Autodesk Inventor part; units mm, degrees
ref_plane "YZ Plane" through (0, 0, 0) normal (1, 0, 0) x (0, 1, 0)
ref_plane "XZ Plane" through (0, 0, 0) normal (0, 1, 0) x (-1, 0, 0)
ref_plane "XY Plane" through (0, 0, 0) normal (0, 0, 1) x (1, 0, 0)
sketch "Szkic1" plane through (0, 0, 0) normal (0, 0, 1) x (1, 0, 0)
  line L0 (-47.736, 26.7667) -> (-47.736, 6.7667)
  line L1 (-47.736, 26.7667) -> (52.264, 26.7667)
  line L2 (52.264, 26.7667) -> (52.264, 6.7667)
  line L3 (52.264, 6.7667) -> (32.264, 6.7667)
  line L4 (32.264, 6.7667) -> (32.264, -48.2333)
  line L5 (32.264, -48.2333) -> (-27.736, -48.2333)
  line L6 (-27.736, -48.2333) -> (-27.736, 6.7667)
  line L7 (-27.736, 6.7667) -> (-47.736, 6.7667)
  circle A0 centre (2.264, -27.7333) radius 19
  arc A1 (-11.0025, -7.7333) -> (-11.0025, -47.7333) centre (2.264, -27.7333) ccw
  line L8 (-11.0025, -47.7333) -> (15.5305, -47.7333)
  arc A2 (15.5305, -47.7333) -> (15.5305, -7.7333) centre (2.264, -27.7333) ccw
  line L9 (15.5305, -7.7333) -> (-11.0025, -7.7333)
  circle A3 centre (2.264, -27.7333) radius 15
  circle A4 centre (-37.736, 16.7667) radius 2
  circle A5 centre (2.264, 16.7667) radius 2
  circle A6 centre (42.264, 16.7667) radius 2
  arc A7 (-23.5765, -30.609) -> (-13.7282, -48.2333) centre (2.264, -27.7333) ccw
  arc A8 (18.2561, -48.2333) -> (28.1044, -30.609) centre (2.264, -27.7333) ccw
  line L10 (-27.736, 6.7667) -> (-23.5765, -30.609)
  line L11 (32.264, 6.7667) -> (28.1044, -30.609)
  line L12 (-7.736, 26.7667) -> (-7.736, 66.7667)
  line L13 (-7.736, 66.7667) -> (12.264, 66.7667)
  line L14 (12.264, 66.7667) -> (12.264, 26.7667)
  circle A9 centre (2.264, 56.7667) radius 2
  point P0 (0, 0)
  point P1 (-16.736, -27.7333)
  point P2 (-11.1711, -41.1683)
  point P3 (15.699, -14.2982)
  point P4 (15.699, -41.1683)
  point P5 (-11.1711, -14.2982)
  point P6 (21.264, -27.7333)
  dimension "d0" = 20
  dimension "d1" = 100
  dimension "d2" = 20
  dimension "d3" = 60
  dimension "d4" = 20
  dimension "d5" = 55
  dimension "d8" = 38
  dimension "d13" = 34.5
  dimension "d14" = 30
  dimension "d15" = 30
  dimension "d24" = 4
  dimension "d25" = 4
  dimension "d26" = 4
  dimension "d29" = 10
  dimension "d30" = 10
  dimension "d31" = 10
  dimension "d32" = 10
  dimension "d33" = 10
  dimension "d34" = 50
  dimension "d42" = 2
  dimension "d47" = 40
  dimension "d48" = 20
  dimension "d49" = 40
  dimension "d50" = 10
  dimension "d51" = 10
  dimension "d52" = 4
extrude "Wyciągnięcie proste1" add sketch "Szkic1" along normal blind 4 contours L1 L2 L3 L11 A8 L5 A7 L10 L7 L0 | L12 L13 L14 L1 | L10 A7 L5 L6 | A8 L11 L4 L5 | A0 | L9 A2 L8 A1 | A3 | A4 | A5 | A6 | A9
extrude "Wyciągnięcie proste2" cut sketch "Szkic1" along normal through all contours A3 | A4 | A5 | A6 | A9
hole "Otwór1" at (2.264, -27.7333, 0) at (21.264, -27.7333, 0) at (-11.1711, -41.1683, 0) at (15.699, -41.1683, 0) at (15.699, -14.2982, 0) at (-11.1711, -14.2982, 0) at (-16.736, -27.7333, 0) direction (0, 0, 1) diameter 5 end through all
extrude "Wyciągnięcie proste3" cut sketch "Szkic1" along normal blind 10 contours L10 A7 L5 L6 | A8 L11 L4 L5
fillet "Zaokrąglenie1" radius 6 8 edges at (-47.736, 6.7667, 2) (-47.736, 26.7667, 2) (52.264, 6.7667, 2) (52.264, 26.7667, 2) (-7.736, 26.7667, 2) (-7.736, 66.7667, 2) (12.264, 26.7667, 2) (12.264, 66.7667, 2)
fillet "Zaokrąglenie2" radius 10 2 edges at (-27.736, 6.7667, 2) (32.264, 6.7667, 2)
fillet "Zaokrąglenie3" radius 8 2 edges at (-13.7282, -48.2333, 2) (18.2561, -48.2333, 2)
equation "\"d2\" = -0.5 * d3 + 0.5 * d1"
equation "\"d34\" = 0.5 * d1"
properties part number "LC_ALU_4mm_Heatbed_Frame_Ball_Screw_Nut_Mounting_Bracket"
Could you check a few things on this model? Use its own coordinates, in mm. A direction names the side the tool comes from. Give positions to 0.01 mm unless a question says otherwise; leave off trailing zeros. Order: outer loops, then holes, each group sorted by start corner. A loop starts at its lowest first (then second) coordinate and runs counter-clockwise, first axis right, second up. Notation, with made-up numbers: (89.25, 25.5) - (109.25, 25.5) arc R12 ccw to (109.25, 41.5) - close; hole circle Ø5 at (-25, -35.75). An arc over 180 degrees is marked (long way). Return JSON: item names as keys, results as strings. Group by question number.
Q1. Thinking about a two-plate mould opening in X: for faces 1 (the face through (52.264, 17, 2)), 2 (the face through (-28, 26.767, 2)), 3 (the face through (-0.99, -13.09, 1.97)), 4 (the face through (3.19, 58.54, 1.97)), which applies, pulls with the +X half, pulls with the -X half, needs draft (parallel to the pull), parting line crosses it, or undercut?
Q2. Which directions (+Z, -Z, +X, -X, +Y, -Y) give clear straight access to the entire face, cutting with the end or side of a thin tool? Please do faces 5 (the face through (-39.323, 17.984, 1.972)), 6 (the face through (44, 6.767, 2)), 7 (the face through (-7.736, 47, 2)).
Q3. Suppose I cut it at B-B, the plane x = 8.5. Please give me the cut outline in (y, z), and give its area (3 significant figures).
Q4. Will these pins go through, and if not, where does the flat tip stop? pin 1 Ø3.5 at (x, y) = (-37.74, 16.77) entering from +Z; pin 2 Ø2 at (y, z) = (47.5, 2) entering from -X; pin 3 Ø6.5 at (x, y) = (2.26, 16.77) entering from -Z; pin 4 Ø2 at (y, z) = (4, 2) entering from -X.
Q5. Suppose I cut it at C-C, the plane y = 36.5. Please give me the cut outline in (x, z), and give its area (3 significant figures).
Q6. Please list where these lines run through material, in increasing order: line 1 along Y through (x, z) = (2.5, 2.35); line 2 along Y through (x, z) = (-38, 0.65); line 3 along Y through (x, z) = (-11, 3.4). Write a range as [from, to].
Q7. Suppose I cut it at D-D, the plane z = 1.5. State how many separate pieces and enclosed holes the cut face has, and give its area (3 significant figures).
Q8. Suppose I cut it at A-A, the plane y = -33. Please give me the cut outline in (x, z), and give its area (3 significant figures).
Resolved:
{
 "1": {"face 1": "pulls with the +X half", "face 2": "needs draft", "face 3": "undercut", "face 4": "undercut"},
 "2": {"face 5": "+Z, -Z", "face 6": "+Z, -Z, +X, -Y", "face 7": "+Z, -Z, -X, +Y"},
 "3": {"outline": "(-48.23, 0) - (-41.38, 0) - (-41.38, 4) - (-48.23, 4) - close; (-14.09, 0) - (66.33, 0) - (66.33, 4) - (-14.09, 4) - close", "area": "349 mm2"},
 "4": {"pin 1": "passes through", "pin 2": "stops at x = -7.74", "pin 3": "stops at z = 0", "pin 4": "stops at x = -31.01"},
 "5": {"outline": "(-7.74, 0) - (12.26, 0) - (12.26, 4) - (-7.74, 4) - close", "area": "80.0 mm2"},
 "6": {"line 1": "y = [-48.23, -42.73], [-12.74, 14.78], [18.75, 54.78], [58.75, 66.77]", "line 2": "y = [6.77, 14.78], [18.75, 26.77]", "line 3": "y = [-48.23, -43.66], [-38.67, -34.74], [-20.73, -16.79], [-11.8, 27.43]"},
 "7": {"separate pieces": "1", "enclosed holes": "11", "area": "4,800 mm2"},
 "8": {"outline": "(-23.2, 0) - (-11.78, 0) - (-11.78, 4) - (-23.2, 4) - close; (16.31, 0) - (27.72, 0) - (27.72, 4) - (16.31, 4) - close", "area": "91.3 mm2"}
}
